The listing builds one solid part. Answer for the finished solid, in the listing's coordinates (mm). A direction names the side the tool comes from. Give positions to 0.01 mm unless a question says otherwise; leave off trailing zeros. Write each loop counter-clockwise with the first axis right and the second up, starting at its lowest first coordinate (ties: lowest second). Pieces come first, ordered by that corner, then holes. Notation, with made-up numbers: (45.25, 54.25) - (98.25, 54.25) arc R31 cw to (98.25, 93.25) - close; hole circle Ø9 at (50, 25). An arc over 180 degrees is marked (long way). Write each question's results on one line, items separated by ' | '. Start each with the question number.
Q1. Section D-D (z = 4.5) is taken. Determine the outline of the cut face in (x, y), plus the area to 3 significant figures.
Q2. Section C-C (y = 3) is taken. Determine the outline of the cut face in (x, z).
Q3. Section A-A (z = 18) is taken. Determine the outline of the cut face in (x, y).
Q4. For faces 1 (the face through (10, 14, 10)), 2 (the face through (30.07, 30.74, 24.65)), 3 (the face through (0, 45, 5)), determine the directions among +Z, -Z, +X, -X, +Y, -Y from which every point of the face is accessible in a straight line to the end or side of a thin tool.
Q5. Section B-B (x = 32.5) is taken. Determine the outline of the cut face in (y, z).
Q6. Find the intervals of material crossed by probe 1 along Y at (x, z) = (18.5, 35.5); probe 2 along Y at (x, z) = (23.5, 11); probe 3 along X at (y, z) = (35.5, 45.5), in increasing order.
Q7. Flat-ended cylindrical pins translate along their axes: pin 1 Ø15 at (x, y) = (16.5, 24) entering from -Z (3 decimals); pin 2 Ø1.5 at (y, z) = (1.5, 20.5) entering from +X; pin 3 Ø1 at (x, z) = (22.5, 7) entering from +Y; pin 4 Ø3.5 at (x, z) = (44, 7.5) entering from -Y. Find the tip coordinate at first contact, or state that the pin passes through.
```python
from build123d import *

# Parameters (mm, degrees)
BOSS_EXTRUDE1_DEPTH = 10
BOSS_EXTRUDE2_DEPTH = 40
BOSS_EXTRUDE3_DEPTH = 40


with BuildPart() as part:
    # Sketch1 → Boss-Extrude1 (new body)
    with BuildSketch(Plane.XY):
        with BuildLine():
            Line((0, 46), (0, 43))
            ThreePointArc((0, 43), (30.405591591, 30.405591591), (43, 0))
            Line((43, 0), (46, 0))
            ThreePointArc((46, 0), (32.526911935, 32.526911935), (0, 46))
        make_face()
    extrude(amount=BOSS_EXTRUDE1_DEPTH)



with BuildPart() as body_2:
    # Sketch3 → Boss-Extrude2 (new body)
    with BuildSketch(Plane.XY.offset(10)):
        with BuildLine():
            Line((0, 46), (-3, 46))
            ThreePointArc((-3, 46), (9.101351514, 9.101351514), (46, -3))
            Line((46, -3), (46, 0))
            Line((46, 0), (43, 0))
            ThreePointArc((43, 0), (12.594408409, 12.594408409), (0, 43))
            Line((0, 43), (0, 46))
        make_face()
    extrude(amount=BOSS_EXTRUDE2_DEPTH)


with BuildPart() as part_1:
    add(part.part)

    add(body_2.part)  # Boss-Extrude3 merges body 2
    # Sketch4 → Boss-Extrude3 (add)
    with BuildSketch(Plane.XY.offset(10)):
        with BuildLine():
            Line((0, 46), (0, 43))
            ThreePointArc((0, 43), (30.405591591, 30.405591591), (43, 0))
            Line((43, 0), (46, 0))
            ThreePointArc((46, 0), (32.526911935, 32.526911935), (0, 46))
        make_face()
    extrude(amount=BOSS_EXTRUDE3_DEPTH)


solid = part_1.part
```
Answers below:
1) outline: (0, 43) arc R43 cw to (43, 0) - (46, 0) arc R46 ccw to (0, 46) - close | area: 210 mm2
2) outline: (16.79, 10) - (27.22, 10) - (27.22, 50) - (16.79, 50) - close; (42.9, 0) - (45.9, 0) - (45.9, 50) - (42.9, 50) - close
3) outline: (-3, 46) arc R43 ccw to (46, -3) - (46, 0) arc R46 ccw to (0, 46) - close; hole (0, 43) arc R43 ccw to (43, 0) arc R43 ccw to start
4) face 1: -Z, -X, -Y | face 2: +Z, -Z | face 3: -Z, -X, +Y, -Y
5) outline: (-2.92, 10) - (1.3, 10) - (1.3, 50) - (-2.92, 50) - close; (28.16, 0) - (32.55, 0) - (32.55, 50) - (28.16, 50) - close
6) probe 1: y = 1.99 to 7.66, 38.82 to 42.12 | probe 2: y = -0.4 to 4.68, 36.01 to 39.54 | probe 3: x = -3.31 to 0.66, 24.26 to 29.25
7) pin 1: passes through | pin 2: stops at x = 45.99 | pin 3: stops at y = 40.4 | pin 4: stops at y = 0
